Design review of the part built by this model. Coordinates are the model's own, in mm. Give positions to 0.01 mm unless a question says otherwise; leave off trailing zeros. Order: outer loops, then holes, each group sorted by start corner. A loop starts at its lowest first (then second) coordinate and runs counter-clockwise, first axis right, second up. Notation, with made-up numbers: (66, 71.5) -> (77, 71.5) arc R14 ccw to (77, 82.5) -> close; hole circle Ø8 at (26.5, 40.25). An arc over 180 degrees is marked (long way). One line per item, written item: value.
from build123d import *

# Parameters (mm, degrees)
F1_DEPTH = 311.15


with BuildPart() as f1:
    # F0 (on Front) → F1 (new body)
    with BuildSketch(Plane.XZ):
        with BuildLine():
            Line((-49.8280417436, 58.7375), (49.8280417436, 58.7375))
            ThreePointArc((49.8280417436, 58.7375), (36.7198515553, 67.7095277786), (22.05, 73.801931887))
            Line((22.05, 73.801931887), (22.05, 71.7951364665))
            ThreePointArc((22.05, 71.7951364665), (18.9376310607, 68.7972416683), (16.0584178523, 72.0197166389))
            Line((16.0584178523, 72.0197166389), (16.0584178523, 75.3329600263))
            ThreePointArc((16.0584178523, 75.3329600263), (-0.00173326, 77.0254999805), (-16.0618081837, 75.3322372436))
            Line((-16.0618081837, 75.3322372436), (-16.0618081837, 72.0610493636))
            ThreePointArc((-16.0618081837, 72.0610493636), (-16.0529534998, 71.9282239397), (-16.05, 71.7951364665))
            ThreePointArc((-16.05, 71.7951364665), (-19.05, 68.7951364665), (-22.05, 71.7951364665))
            Line((-22.05, 71.7951364665), (-22.05, 73.801931887))
            ThreePointArc((-22.05, 73.801931887), (-36.7198515553, 67.7095277787), (-49.8280417436, 58.7375))
        make_face()
    extrude(amount=F1_DEPTH)


solid = f1.part
Item 1: To check wall thickness, follow line 1 along X through (y, z) = (-239, 71.5); line 2 along Z through (x, y) = (1, -177.5); line 3 along Z through (x, y) = (28, -24). State the ranges of each line that lie inside material, in increasing order. Write a range as from..to.
Returned:
line 1: -28.65..-22.04, -16.06..16.06, 22.04..28.65
line 2: 58.74..77.02
line 3: 58.74..71.76
Item 2: Add section C-C on z = 63. Give the boundary of the cut face in (x, y), plus the area to 3 significant figures.
Returned:
outline: (-44.32, -311.15) -> (44.32, -311.15) -> (44.32, 0) -> (-44.32, 0) -> close
area: 27,600 mm²
Item 3: Draft analysis for pull direction X (two halves, no side actions). For faces 1 (the flat face through (-1, -153, 58.738)), 2 (the cylindrical face through (0.225, -153.397, 77.025)), 3 (the cylindrical face through (19.005, -153.397, 68.795)), 4 (the cylindrical face through (-36.524, -153.397, 67.815)), state which applies: pulls with the +X half, pulls with the -X half, needs draft (parallel to the pull), parting line crosses it, or undercut.
Returned:
face 1: needs draft
face 2: parting line crosses it
face 3: undercut
face 4: pulls with the -X half
Item 4: Add section A-A on y = -243.5. Give the boundary of the cut face in (x, z).
Returned:
outline: (-49.83, 58.74) -> (49.83, 58.74) arc R77.03 ccw to (22.05, 73.8) -> (22.05, 71.8) arc R3 cw (long way) to (16.06, 72.02) -> (16.06, 75.33) arc R77.03 ccw to (-16.06, 75.33) -> (-16.06, 72.06) arc R3 cw (long way) to (-22.05, 71.8) -> (-22.05, 73.8) arc R77.03 ccw to start
Item 5: Clearance check with flat-ended pins moving along their axes: P1, Ø2, axis at x = -18, y = -84.5, coming from the +Z side; P2, Ø10, axis at x = 37.5, y = -64, coming from the +Z side; P3, Ø12, axis at x = -8.5, y = -95, coming from the +Z side. State where each tip first meets the part, or that it passes through.
Returned:
P1: z = 69.6
P2: z = 69.83
P3: z = 76.98
Item 6: Add section B-B on x = 19.05. Give the boundary of the cut face in (y, z), plus the area to 3 significant figures.
Returned:
outline: (-311.15, 58.74) -> (0, 58.74) -> (0, 68.8) -> (-311.15, 68.8) -> close
area: 3,130 mm²
